Input: part model. Units: mm. Frame: model coordinates. Give positions to 0.01 mm unless a question says otherwise; leave off trailing zeros. Loops run counter-clockwise (first coordinate to the right, second up) from the corner with the lowest first, then second, coordinate; pieces in that order, holes last. Notation, with made-up numbers: M -1.75,83 L 16.25,83 A30 cw 16.25,119 Z; hole C 72,-17 d7. An arc over 180 degrees is marked long. One line per item, written item: value. Start each with the question number.
(1) Pin query (flat end, axial travel): P1, Ø1, axis at y = -82.5, z = 2.5, coming from the -X side; P2, Ø1.5, axis at y = -63, z = 1.5, coming from the +X side; P3, Ø1.2, axis at x = 301, z = 1.5, coming from the +Y side; P4, Ø6, axis at x = 319.5, y = 7, coming from the -Z side. Return the tip coordinate at first contact, or that it passes through.
(2) Section C-C on y = -11. Output: boundary loops of the cut face in (x, z).
(3) Ray query, line 1 along Y through (x, z) = (303.5, 0.65); line 2 along Y through (x, z) = (307.5, 3.65); line 3 along X through (y, z) = (-22, 2.7). Return the intervals inside material, ascending. Write a range as from..to.
(4) Section B-B on x = 346. Output: boundary loops of the cut face in (y, z).
(5) Section D-D on x = 335. Output: boundary loops of the cut face in (y, z), plus the area to 3 significant figures.
(6) Section A-A on y = 2. Output: boundary loops of the cut face in (x, z).
```python
from build123d import *

# Parameters (mm, degrees)
SKETCH_1_R      = 5.03
EXTRUDE_1_DEPTH = 4


with BuildPart() as part:
    # 草图1 → 凸台-拉伸1 (new body)
    with BuildSketch(Plane.XY):
        with BuildLine():
            Line((298.542857143, -51.645714286), (302.542857143, -51.645714286))
            Line((302.542857143, -51.645714286), (302.542857143, -53.644175919))
            Line((302.542857143, -53.644175919), (305.242857143, -53.644175919))
            Line((305.242857143, -53.644175919), (305.242857143, -51.645714286))
            Line((305.242857143, -51.645714286), (307.942857143, -51.645714286))
            Line((307.942857143, -51.645714286), (307.942857143, -48.645714286))
            Line((307.942857143, -48.645714286), (305.242857143, -48.645714286))
            Line((305.242857143, -48.645714286), (305.242857143, -46.647252653))
            Line((305.242857143, -46.647252653), (302.542857143, -46.647252653))
            Line((302.542857143, -46.647252653), (302.542857143, -48.645714286))
            Line((302.542857143, -48.645714286), (298.542857143, -48.645714286))
            Line((298.542857143, -48.645714286), (298.542857143, -39.145714286))
            Line((298.542857143, -39.145714286), (294.542857143, -39.145714286))
            Line((294.542857143, -39.145714286), (294.542857143, -31.145714286))
            Line((294.542857143, -31.145714286), (298.542857143, -31.145714286))
            Line((298.542857143, -31.145714286), (298.542857143, -21.645714286))
            Line((298.542857143, -21.645714286), (302.542857143, -21.645714286))
            Line((302.542857143, -21.645714286), (302.542857143, -23.644175919))
            Line((302.542857143, -23.644175919), (305.242857143, -23.644175919))
            Line((305.242857143, -23.644175919), (305.242857143, -21.645714286))
            Line((305.242857143, -21.645714286), (307.942857143, -21.645714286))
            Line((307.942857143, -21.645714286), (307.942857143, -18.645714286))
            Line((307.942857143, -18.645714286), (305.242857143, -18.645714286))
            Line((305.242857143, -18.645714286), (305.242857143, -16.647252653))
            Line((305.242857143, -16.647252653), (302.542857143, -16.647252653))
            Line((302.542857143, -16.647252653), (302.542857143, -18.645714286))
            Line((302.542857143, -18.645714286), (298.542857143, -18.645714286))
            Line((298.542857143, -18.645714286), (298.542857143, -9.145714286))
            Line((298.542857143, -9.145714286), (294.542857143, -9.145714286))
            Line((294.542857143, -9.145714286), (294.542857143, -1.145714286))
            Line((294.542857143, -1.145714286), (298.542857143, -1.145714286))
            Line((298.542857143, -1.145714286), (298.542857143, -0.145714286))
            Line((298.542857143, -0.145714286), (298.542857143, 14.854285714))
            Line((298.542857143, 14.854285714), (324.186090726, 17.3685065))
            ThreePointArc((324.186090726, 17.3685065), (357.743319291, 28.408646086), (378.542857143, -0.145714286))
            Line((378.542857143, -0.145714286), (378.542857143, -52.102236025))
            Line((378.542857143, -52.102236025), (313.542857143, -100.145714286))
            Line((313.542857143, -100.145714286), (298.542857143, -100.145714286))
            Line((298.542857143, -100.145714286), (298.542857143, -81.645714286))
            Line((298.542857143, -81.645714286), (302.542857143, -81.645714286))
            Line((302.542857143, -81.645714286), (302.542857143, -83.644175919))
            Line((302.542857143, -83.644175919), (305.242857143, -83.644175919))
            Line((305.242857143, -83.644175919), (305.242857143, -81.645714286))
            Line((305.242857143, -81.645714286), (307.942857143, -81.645714286))
            Line((307.942857143, -81.645714286), (307.942857143, -78.645714286))
            Line((307.942857143, -78.645714286), (305.242857143, -78.645714286))
            Line((305.242857143, -78.645714286), (305.242857143, -76.647252653))
            Line((305.242857143, -76.647252653), (302.542857143, -76.647252653))
            Line((302.542857143, -76.647252653), (302.542857143, -78.645714286))
            Line((302.542857143, -78.645714286), (298.542857143, -78.645714286))
            Line((298.542857143, -78.645714286), (298.542857143, -69.145714286))
            Line((298.542857143, -69.145714286), (294.542857143, -69.145714286))
            Line((294.542857143, -69.145714286), (294.542857143, -61.145714286))
            Line((294.542857143, -61.145714286), (298.542857143, -61.145714286))
            Line((298.542857143, -61.145714286), (298.542857143, -51.645714286))
        make_face()
        with Locations((348.542857143, -0.145714286)):
            Circle(SKETCH_1_R, mode=Mode.SUBTRACT)
    extrude(amount=EXTRUDE_1_DEPTH)


solid = part.part
```
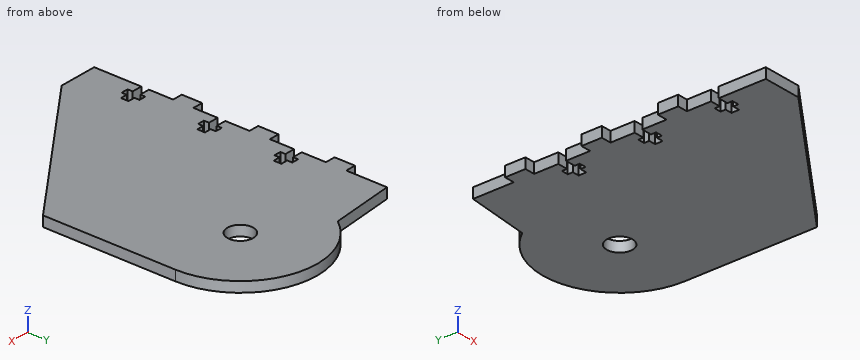
Output values:
1. P1: stops at x = 298.54
1. P2: stops at x = 364.81
1. P3: stops at y = 15.15
1. P4: stops at z = 0
2. outline: M 298.54,0 L 378.54,0 L 378.54,4 L 298.54,4 Z
3. line 1: y = -100.15..-83.64, -76.65..-53.64, -46.65..-23.64, -16.65..15.34
3. line 2: y = -100.15..-81.65, -78.65..-51.65, -48.65..-21.65, -18.65..15.73
3. line 3: x = 298.54..302.54, 305.24..378.54
4. outline: M -76.16,0 L -4.49,0 L -4.49,4 L -76.16,4 Z; M 4.19,0 L 29.75,0 L 29.75,4 L 4.19,4 Z
5. outline: M -84.29,0 L 26.62,0 L 26.62,4 L -84.29,4 Z
5. area: 444 mm²
6. outline: M 298.54,0 L 343.99,0 L 343.99,4 L 298.54,4 Z; M 353.09,0 L 378.47,0 L 378.47,4 L 353.09,4 Z
